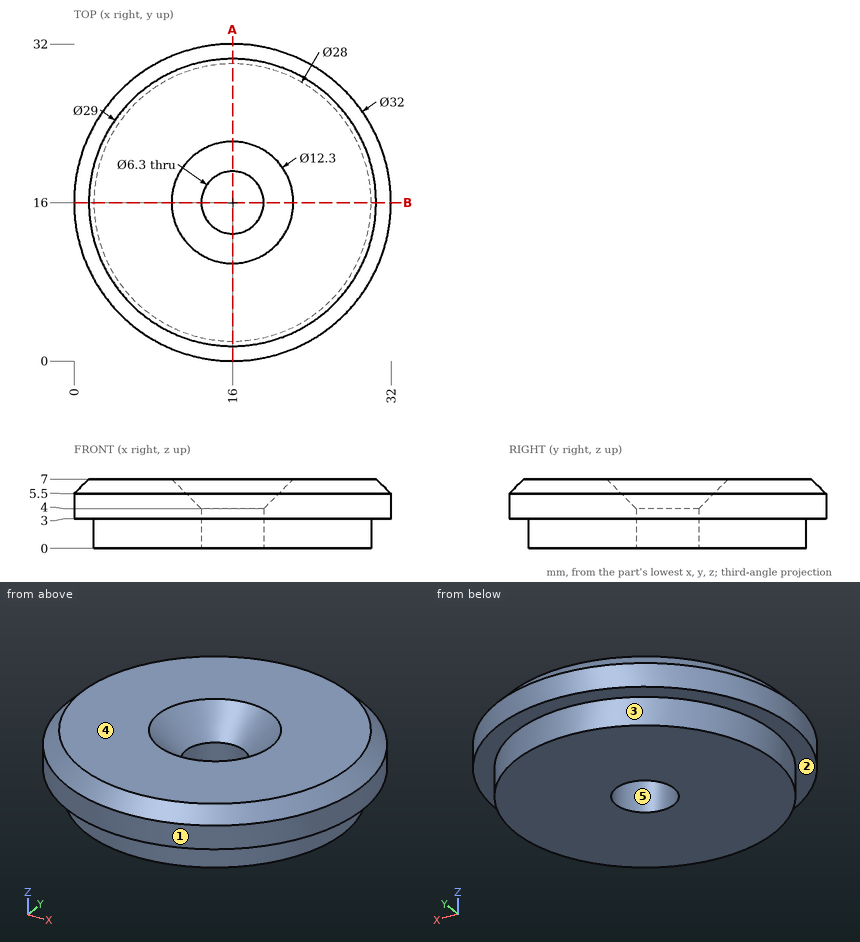
Design review of the part shown in the three views and the two pictorial views. Dimensions are in mm from the part's minimum x, y and z. A direction names the side the tool comes from. Coordinates: 2 decimals unless noted, no trailing zeros. Order: outer loops, then holes, each group sorted by start corner. A loop starts at its lowest first (then second) coordinate and runs counter-clockwise, first axis right, second up.
Item 1: The part is to be moulded in two halves that separate along Y. For the marked faces 3, 4 and 5, say which applies: pulls with the +Y half, pulls with the -Y half, needs draft (parallel to the pull), parting line crosses it, or undercut.
Item 2: For line 1 (Y direction, x = 16, z = 2.75); line 2 (X direction, y = 17.5, z = 4.25); line 3 (X direction, y = 15, z = 3.5), list the stretches that pass through material, from the lowest coordinate up.
Item 3: Take a section at A-A, the plane x = 16. Write out the cut boundary in (y, z).
Item 4: For pin 1 Ø1.5 at (y, z) = (15.5, 4) entering from +X; pin 2 Ø2 at (y, z) = (11.5, 1.5) entering from +X; pin 3 Ø2 at (y, z) = (10.5, 4.5) entering from +X; pin 4 Ø5.5 at (x, y) = (16, 16) entering from -Z, all flat-tipped, find the tip position at first contact; note any pin that passes through.
Item 5: For the marked faces 1 and 2, list the 3-axis set-ups (+Z, -Z, +X, -X, +Y, -Y) from which the entire face can be reached by the end or side of a thin tool; tool diameter is ignored.
The answers:
1. face 3: parting line crosses it
1. face 4: needs draft
1. face 5: undercut
2. line 1: y = 2 to 12.85, 19.15 to 30
2. line 2: x = 0.07 to 12.95, 19.05 to 31.93
2. line 3: x = 0.03 to 13.01, 18.99 to 31.97
3. outline: (0, 3) - (2, 3) - (2, 0) - (12.85, 0) - (12.85, 4) - (9.85, 7) - (1.5, 7) - (0, 5.5) - close; (19.15, 0) - (30, 0) - (30, 3) - (32, 3) - (32, 5.5) - (30.5, 7) - (22.15, 7) - (19.15, 4) - close
4. pin 1: stops at x = 32
4. pin 2: stops at x = 29.56
4. pin 3: stops at x = 31.35
4. pin 4: passes through
5. face 1: +Z, -Z
5. face 2: -Z
